For this review, take the finished solid that the model builds, in its own axes (mm). Face numbers are marked on the shaded views. A direction names the side the tool comes from. Coordinates: 2 decimals unless noted, no trailing zeros. Order: outer loops, then holes, each group sorted by start corner. A loop starts at its lowest first (then second) coordinate and runs counter-clockwise, first axis right, second up. Notation, with made-up numbers: (40.5, 56) -> (95.5, 56) arc R17 cw to (95.5, 84) -> close; hole circle Ø11 at (62.5, 67). An arc over 180 degrees is marked (long way). Write item = value, one per line. Start each with the question number.
1) Insertion check: pin 1 Ø2 at (x, z) = (11, -34) entering from -Y; pin 2 Ø4 at (y, z) = (-9.5, -38.5) entering from +X. Each pin has a flat end and moves straight along its axis. Give the tip position at first contact, or say it passes through.
2) Consider section C-C on x = 9.5. Give the boundary of the cut face in (y, z).
3) Consider section B-B on y = -51.5. Give the boundary of the cut face in (x, z), and give its area (3 significant figures).
4) Machinability: for the marked faces 4 and 5, which of the approach directions +Z, -Z, +X, -X, +Y, -Y give a long, thin tool a straight path to every point of the face, cutting with its end or side? Answer none if there is none.
5) Consider section D-D on z = -3. Give the boundary of the cut face in (x, y).
6) Draft analysis for pull direction Z (two halves, no side actions). For the marked faces 1, 2 and 3, state which applies: +Z half, -Z half, draft (parallel to the pull), parting line (faces both ways), or undercut.
7) Wall thickness on probe 1 along Z at (x, y) = (3.5, -55.5); probe 2 along Y at (x, z) = (13, -53); probe 3 along X at (y, z) = (-16.5, -32.5): over which ranges is each line inside the solid? List them lowest first. Write a range as [from, to].
8) Consider section A-A on z = -46. Give the boundary of the cut face in (x, y).
from build123d import *

# Parameters (mm, degrees)
SKETCH1_W           = 61.34
SKETCH1_H           = 76.58
SKETCH1_W_2         = 53.34
SKETCH1_H_2         = 68.58
BOSS_EXTRUDE1_DEPTH = 15
SKETCH2_W           = 61.34
SKETCH2_H           = 76.58
BOSS_EXTRUDE2_DEPTH = 5
SKETCH4_W           = 19.05
SKETCH4_H           = 53.34
CUT_EXTRUDE2_DEPTH  = 21
SKETCH5_W           = 12
SKETCH5_H           = 4
BOSS_EXTRUDE3_DEPTH = 15


with BuildPart() as part:
    # Sketch1 → Boss-Extrude1 (new body)
    with BuildSketch(Plane(origin=(0, 0, 0), x_dir=(0, 0, -1), z_dir=(1, 0, 0))):
        with Locations((26.67, -34.29)):
            Rectangle(SKETCH1_W, SKETCH1_H)
        with Locations((26.67, -34.29)):
            Rectangle(SKETCH1_W_2, SKETCH1_H_2, mode=Mode.SUBTRACT)
    extrude(amount=BOSS_EXTRUDE1_DEPTH)

    # Sketch2 → Boss-Extrude2 (add)
    with BuildSketch(Plane.ZY):
        with Locations((-26.67, -34.29)):
            Rectangle(SKETCH2_W, SKETCH2_H)
    extrude(amount=BOSS_EXTRUDE2_DEPTH)

    # Sketch4 → Cut-Extrude2 (cut)
    with BuildSketch(Plane(origin=(0, -72.58, 0), x_dir=(-1, 0, 0), z_dir=(0, -1, 0))):
        with Locations((-9.525, 26.67)):
            Rectangle(SKETCH4_W, SKETCH4_H)
    extrude(amount=-CUT_EXTRUDE2_DEPTH, mode=Mode.SUBTRACT)

    # Sketch5 → Boss-Extrude3 (add)
    with BuildSketch(Plane(origin=(0, 0, 0), x_dir=(0, 0, -1), z_dir=(1, 0, 0))):
        with Locations((47.34, -70.58)):
            Rectangle(SKETCH5_W, SKETCH5_H)
    extrude(amount=BOSS_EXTRUDE3_DEPTH)


solid = part.part
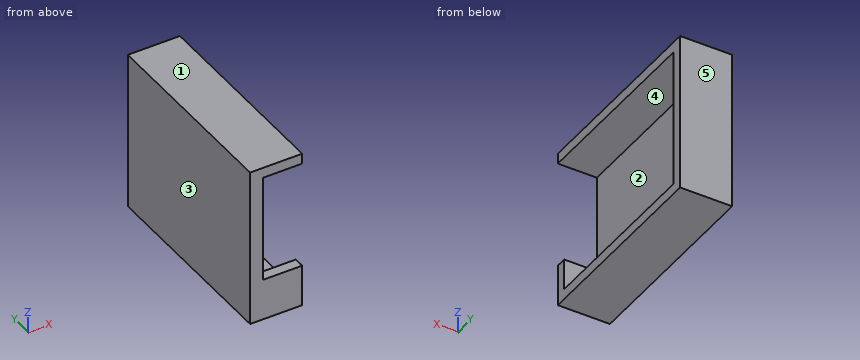
Answer sheet:
q1.pin_1 = 0
q1.pin_2 = 0
q2.outline = (-72.58, -57.34) -> (4, -57.34) -> (4, 4) -> (-72.58, 4) -> (-72.58, 0) -> (0, 0) -> (0, -53.34) -> (-68.58, -53.34) -> (-68.58, -41.34) -> (-72.58, -41.34) -> close
q3.outline = (-5, -57.34) -> (15, -57.34) -> (15, -53.34) -> (0, -53.34) -> (0, 0) -> (15, 0) -> (15, 4) -> (-5, 4) -> close
q3.area = 427 mm2
q4.face_4 = +X, -Y
q4.face_5 = +Z, -Z, +X, -X, +Y
q5.outline = (-5, -72.58) -> (0, -72.58) -> (0, 0) -> (15, 0) -> (15, 4) -> (-5, 4) -> close
q6.face_1 = +Z half
q6.face_2 = undercut
q6.face_3 = draft
q7.probe_1 = [-57.34, -53.34], [0, 4]
q7.probe_2 = [-72.58, -68.58], [0, 4]
q7.probe_3 = [-5, 0]
q8.outline = (-5, -72.58) -> (15, -72.58) -> (15, -68.58) -> (0, -68.58) -> (0, 0) -> (15, 0) -> (15, 4) -> (-5, 4) -> close
